The model under review builds one solid part; all positions refer to its coordinate system, in mm. A direction names the side the tool comes from. Round coordinates to 2 decimals unless told otherwise and drop trailing zeros. Loops run counter-clockwise (first coordinate to the right, second up) from the corner with the lowest first, then second, coordinate; pieces in that order, holes last. Notation, with made-up numbers: (-10, 58) -> (19, 58) arc R25 ccw to (19, 78) -> close; hole circle Ø6 at (-21, 18). An arc over 180 degrees is marked (long way). Use CSV: the item, a comma, the result in double quotes. Start each with the question number.
```python
from build123d import *


with BuildPart() as part:
    # Sketch1 → Revolve1 (revolve)
    with BuildSketch(Plane.XY, mode=Mode.PRIVATE) as revolve1_sk:
        with BuildLine():
            Line((-11, 4.08), (-11, 0))
            Line((-11, 0), (27, 0))
            Line((27, 0), (27, 2.3865))
            Line((27, 2.3865), (26.3865, 3))
            Line((26.3865, 3), (17.2, 3))
            ThreePointArc((17.2, 3), (17.058578644, 3.058578644), (17, 3.2))
            Line((17, 3.2), (17, 5.5))
            Line((17, 5.5), (16.5, 6))
            Line((16.5, 6), (0.2, 6))
            Line((0.2, 6), (0, 5.8))
            Line((0, 5.8), (0, 5.2))
            ThreePointArc((0, 5.2), (-0.058578644, 5.058578644), (-0.2, 5))
            Line((-0.2, 5), (-10.08, 5))
            Line((-10.08, 5), (-11, 4.08))
        make_face()
    revolve(revolve1_sk.sketch.rotate(Axis((-11, 0, 0), (1, 0, 0)), 270), axis=Axis((-11, 0, 0), (1, 0, 0)))


solid = part.part
```
1. Take a section at C-C, the plane x = 7. Give the boundary of the cut face in (y, z).
2. For faces 3 (the face through (0, 5, 2)), 4 (the face through (27, 0, 0)), 5 (the face through (21.73, 0.9, -2.86)), list the 3-axis set-ups (+Z, -Z, +X, -X, +Y, -Y) from which the entire face can be reached by the end or side of a thin tool; tool diameter is ignored.
3. Take a section at D-D, the plane x = -8. Give the boundary of the cut face in (y, z).
4. For line 1 along X through (y, z) = (-4.75, 2.25); line 2 along X through (y, z) = (-0.25, 3.5); line 3 along Z through (x, y) = (8, -3), list the stretches that pass through material, from the lowest coordinate up. Write a range as from..to.
5. The part is to be moulded in two halves that separate along Z. For faces 1 (the face through (17, -2.4, 2.4)), 2 (the face through (-5.21, -4.88, 1.08)), say which applies: pulls with the +Z half, pulls with the -Z half, needs draft (parallel to the pull), parting line crosses it, or undercut.
6. Take a section at A-A, the plane y = 0. Give the boundary of the cut face in (x, z).
7. Clearance check with flat-ended pins moving along their axes: P1, Ø6, axis at y = 4.5, z = 0.5, coming from the -X side; P2, Ø2, axis at x = 7.5, y = -2.5, coming from the -Z side; P3, Ø2, axis at y = -3.5, z = 4, coming from the +X side; P4, Ø3, axis at x = -0.5, y = -1.5, coming from the +Z side. State where each tip first meets the part, or that it passes through.
Results:
1,outline,"circle Ø12 at (0, 0)"
2,face 3,"-X"
2,face 4,"+Z, -Z, +X, +Y, -Y"
2,face 5,"+X"
3,outline,"circle Ø10 at (0, 0)"
4,line 1,"0..17"
4,line 2,"-11..17"
4,line 3,"-5.2..5.2"
5,face 1,"needs draft"
5,face 2,"parting line crosses it"
6,outline,"(-11, -4.08) -> (-10.08, -5) -> (-0.2, -5) arc R0.2 cw to (0, -5.2) -> (0, -5.8) -> (0.2, -6) -> (16.5, -6) -> (17, -5.5) -> (17, -3.2) arc R0.2 cw to (17.2, -3) -> (26.39, -3) -> (27, -2.39) -> (27, 2.39) -> (26.39, 3) -> (17.2, 3) arc R0.2 cw to (17, 3.2) -> (17, 5.5) -> (16.5, 6) -> (0.2, 6) -> (0, 5.8) -> (0, 5.2) arc R0.2 cw to (-0.2, 5) -> (-10.08, 5) -> (-11, 4.08) -> close"
7,P1,"x = -11"
7,P2,"z = -5.81"
7,P3,"x = 17"
7,P4,"z = 6"
